```python
from build123d import *

# Parameters (mm, degrees)
SKETCH1_W           = 25
SKETCH1_H           = 50
BOSS_EXTRUDE1_DEPTH = 6
SKETCH2_R           = 9
CUT_EXTRUDE1_DEPTH  = 36.619307578


with BuildPart() as part:
    # Sketch1 → Boss-Extrude1 (new body)
    with BuildSketch(Plane.XY):
        with Locations((-3.289473684, -6.359649123)):
            Rectangle(SKETCH1_W, SKETCH1_H)
    extrude(amount=BOSS_EXTRUDE1_DEPTH)

    # Sketch2 → Cut-Extrude1 (cut, through all)
    with BuildSketch(Plane.XY.offset(6)):
        with Locations((-3.442256095, 8.409317212)):
            Circle(SKETCH2_R)
        with Locations((-3.442256095, -18.590682788)):
            Circle(SKETCH2_R)
        with BuildLine():
            Line((7.19958983, -3.041196046), (7.161332442, -6.790420083))
            ThreePointArc((7.161332442, -6.790420083), (4.414711412, -9.481553819), (1.723577676, -6.734932789))
            Line((1.723577676, -6.734932789), (1.761835064, -2.985708753))
            ThreePointArc((1.761835064, -2.985708753), (4.508456094, -0.294575016), (7.19958983, -3.041196046))
        make_face()
    extrude(amount=-CUT_EXTRUDE1_DEPTH, mode=Mode.SUBTRACT)


solid = part.part
```
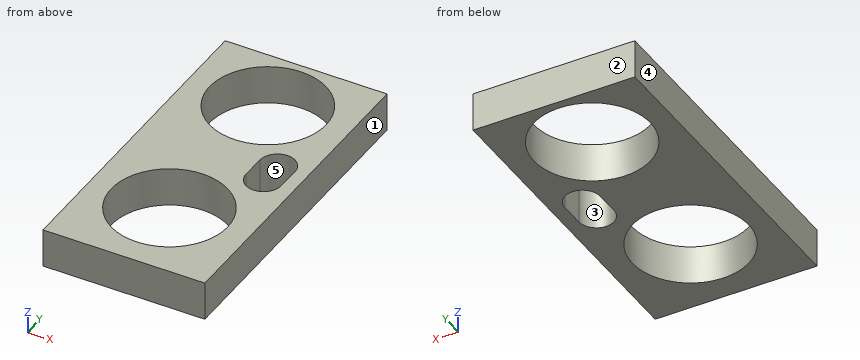
For this review, take the finished solid that the model builds, in its own axes (mm). Face numbers are marked on the shaded views. A direction names the side the tool comes from. Give positions to 0.01 mm unless a question says otherwise; leave off trailing zeros. Loops run counter-clockwise (first coordinate to the right, second up) from the corner with the lowest first, then second, coordinate; pieces in that order, holes last. Notation, with made-up numbers: M 36.5,60.5 L 58.5,60.5 A36 ccw 58.5,95.5 Z; hole C 8,4 d5. An arc over 180 degrees is marked long. One line per item, written item: value. Start each with the question number.
Q1. Machinability: for the marked faces 4 and 5, which of the approach directions +Z, -Z, +X, -X, +Y, -Y give a long, thin tool a straight path to every point of the face, cutting with its end or side? Answer none if there is none.
Q2. For L1, parallel to Y at x = -2.75, z = 0.75; L2, parallel to Y at x = -5, z = 5.25; L3, parallel to X at y = 4.5, z = 5, list the stretches that pass through material, from the lowest coordinate up.
Q3. Clearance check with a flat-ended pin moving along its axis: pin 1 Ø2 at (x, y) = (-7.5, -12) entering from +Z. State where the tip first meets the part, or that it passes through.
Q4. Add section D-D (x = -11). Give the boundary of the cut face in (y, z), and give its area (3 significant figures).
Q5. Add section C-C (z = 4.25). Give the boundary of the cut face in (x, y), and give its area (3 significant figures).
Q6. Add section A-A (y = 13). Give the boundary of the cut face in (x, z), and give its area (3 significant figures).
Q7. Add section B-B (x = -6). Give the boundary of the cut face in (y, z), and give its area (3 significant figures).
Q8. Draft analysis for pull direction X (two halves, no side actions). For the marked faces 1, 2 and 3, state which applies: released by +X, released by -X, zero draft, split by the parting line, or undercut.
Reply:
1. face 4: +Z, -Z, -X, +Y, -Y
1. face 5: +Z, -Z
2. L1: -31.36 to -27.56, -9.62 to -0.56, 17.38 to 18.64
2. L2: -31.36 to -27.45, -9.73 to -0.45, 17.27 to 18.64
2. L3: -15.79 to -11.55, 4.66 to 9.21
3. pin 1: through
4. outline: M -31.36,0 L -23.48,0 L -23.48,6 L -31.36,6 Z; M -13.7,0 L 3.52,0 L 3.52,6 L -13.7,6 Z; M 13.3,0 L 18.64,0 L 18.64,6 L 13.3,6 Z
4. area: 183 mm²
5. outline: M -15.79,-31.36 L 9.21,-31.36 L 9.21,18.64 L -15.79,18.64 Z; hole C -3.44,-18.59 d18; hole C -3.44,8.41 d18; hole M 1.72,-6.73 A2.72 ccw 7.16,-6.79 L 7.2,-3.04 A2.72 ccw 1.76,-2.99 Z
5. area: 697 mm²
6. outline: M -15.79,0 L -11.18,0 L -11.18,6 L -15.79,6 Z; M 4.3,0 L 9.21,0 L 9.21,6 L 4.3,6 Z
6. area: 57.1 mm²
7. outline: M -31.36,0 L -27.22,0 L -27.22,6 L -31.36,6 Z; M -9.96,0 L -0.22,0 L -0.22,6 L -9.96,6 Z; M 17.04,0 L 18.64,0 L 18.64,6 L 17.04,6 Z
7. area: 92.9 mm²
8. face 1: released by +X
8. face 2: zero draft
8. face 3: undercut
